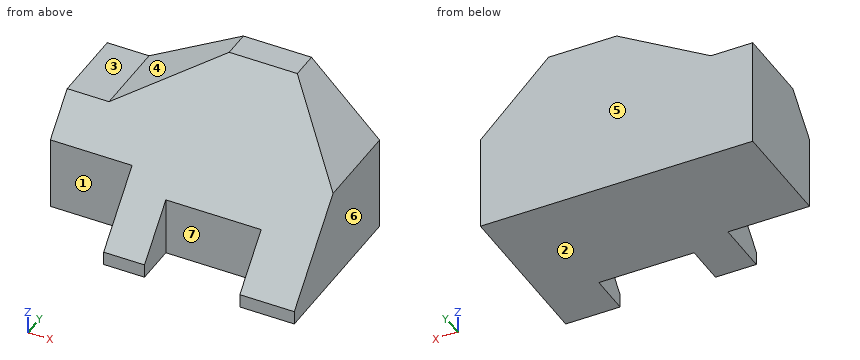
```python
from build123d import *

# Parameters (mm, degrees)
F1_DEPTH = 50
F2_W     = 35
F2_H     = 15
F2_W_2   = 30
F2_H_2   = 20
F3_DEPTH = 60.001
F5_DEPTH = 60.001


with BuildPart() as f1:
    # F0 (on Right) → F1 (new body, symmetric)
    with BuildSketch(Plane.YZ):
        Polygon((0, 5), (0, 0), (60, 0), (60, 60), (50, 60), align=None)
    extrude(amount=F1_DEPTH, both=True)

    # F2 (on face) → F3 (cut, through all)
    with BuildSketch(Plane(origin=(0, 0, 0), x_dir=(1, 0, 0), z_dir=(0, 0, -1))):
        with Locations((12.5, -7.5)):
            Rectangle(F2_W, F2_H)
        with Locations((-35, -10)):
            Rectangle(F2_W_2, F2_H_2)
    extrude(amount=-F3_DEPTH, mode=Mode.SUBTRACT)

    # F4 (on face) → F5 (cut, through all)
    with BuildSketch(Plane(origin=(0, 60, 0), x_dir=(-1, 0, 0), z_dir=(0, 1, 0))):
        Polygon((50, 60), (0, 60), (34.641016, 40), (50, 40), align=None)
        Polygon((-25, 60), (-50, 60), (-50, 35), align=None)
    extrude(amount=-F5_DEPTH, mode=Mode.SUBTRACT)


solid = f1.part
```
The listing builds one solid part. Answer for the finished solid, in the listing's coordinates (mm). Face numbers are marked on the shaded views. A direction names the side the tool comes from. Give positions to 0.01 mm unless a question says otherwise; leave off trailing zeros. Order: outer loops, then holes, each group sorted by start corner. A loop starts at its lowest first (then second) coordinate and runs counter-clockwise, first axis right, second up.
Item 1: The part is cut by section D-D, the plane z = 8. Give the vertices of the cut face in (x, y).
From the geometry:
outline: (-50, 20) - (-20, 20) - (-20, 2.73) - (-5, 2.73) - (-5, 15) - (30, 15) - (30, 2.73) - (50, 2.73) - (50, 60) - (-50, 60) - close
Item 2: The part is cut by section B-B, the plane x = 41.5. Give the vertices of the cut face in (y, z), and give its area (3 significant figures).
From the geometry:
outline: (0, 0) - (60, 0) - (60, 43.5) - (35, 43.5) - (0, 5) - close
area: 1,940 mm2
Item 3: For a pull along X with two mould halves and no side action, classify the marked faces 4, 5, 6 and 7 as pulls with the +X half, pulls with the -X half, needs draft (parallel to the pull), parting line crosses it, or undercut.
From the geometry:
face 4: pulls with the -X half
face 5: needs draft
face 6: pulls with the +X half
face 7: undercut
Item 4: Which of the six approach directions +Z, -Z, +X, -X, +Y, -Y give full straight-line access (tool end or side, diameter ignored) to the marked faces 1, 2 and 3?
From the geometry:
face 1: +Z, -Z, -X, -Y
face 2: -Z, +X, -X, +Y, -Y
face 3: +Z, -X, +Y, -Y
Item 5: Given pin 1 Ø17 at (x, y) = (-39, 51.5) entering from +Z; pin 2 Ø5 at (y, z) = (51, 48) entering from -X; pin 3 Ø10 at (x, y) = (-38, 19.5) entering from +Z, each flat-ended and moving along its own axis, determine where each tip first touches the part or whether it passes through.
From the geometry:
pin 1: stops at z = 42.39
pin 2: stops at x = -25.11
pin 3: stops at z = 31.95
Item 6: Find the intervals of material crossed by probe 1 along X at (y, z) = (7.5, 8.5); probe 2 along Y at (x, z) = (-27, 43.5); probe 3 along Y at (x, z) = (-43.5, 7), in increasing order.
From the geometry:
probe 1: x = -20 to -5, 30 to 50
probe 2: y = 35 to 60
probe 3: y = 20 to 60
Item 7: The part is cut by section C-C, the plane y = 53.5. Give the vertices of the cut face in (x, z).
From the geometry:
outline: (-50, 0) - (50, 0) - (50, 35) - (25, 60) - (0, 60) - (-34.64, 40) - (-50, 40) - close
Item 8: The part is cut by section A-A, the plane y = 6. Give the vertices of the cut face in (x, z).
From the geometry:
outline: (-20, 0) - (-5, 0) - (-5, 11.6) - (-20, 11.6) - close; (30, 0) - (50, 0) - (50, 11.6) - (30, 11.6) - close
